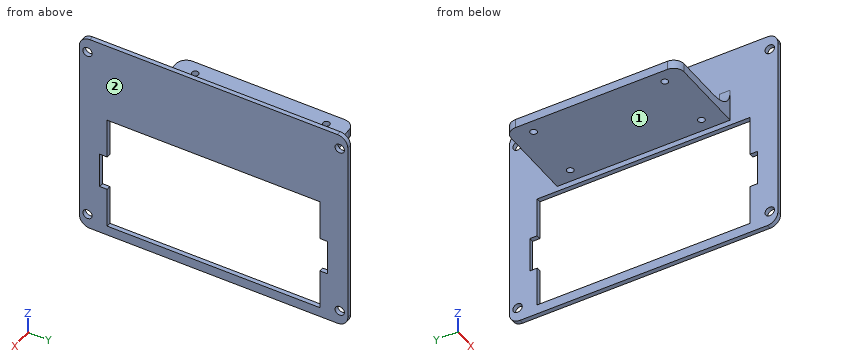
Autodesk Fusion 360 part; units mm, degrees
sketch "Sketch1" plane through (0, 0, 0) normal (1, 0, 0) x (0, 1, 0)
  line L0 (45, 35) -> (-45, 35)
  line L1 (-45, 35) -> (-45, -35)
  line L2 (-45, -35) -> (45, -35)
  line L3 (45, -35) -> (45, 35)
  line L4 (45, 35) -> (-45, -35) construction
  line L5 (-45, 35) -> (45, -35) construction
  line L6 (0, 0) -> (0, -35) construction
  line L7 (39.5, 9.4262) -> (-39.5, 9.4262) construction
  line L8 (-39.5, 9.4262) -> (-39.5, -33.5738) construction
  line L9 (-39.5, -33.5738) -> (39.5, -33.5738) construction
  line L10 (39.5, -33.5738) -> (39.5, 9.4262) construction
  line L11 (39.5, 9.4262) -> (-39.5, -33.5738) construction
  line L12 (-39.5, 9.4262) -> (39.5, -33.5738) construction
  line L13 (35.7, 7.5762) -> (-35.7, 7.5762)
  line L14 (-35.7, 7.5762) -> (-35.7, -31.7238)
  line L15 (-35.7, -31.7238) -> (35.7, -31.7238)
  line L16 (35.7, -31.7238) -> (35.7, 7.5762)
  line L17 (35.7, 7.5762) -> (-35.7, -31.7238) construction
  line L18 (-35.7, 7.5762) -> (35.7, -31.7238) construction
  circle A0 centre (42.2913, -30.0813) radius 1.575
  line L19 (0, 0) -> (10.5805, 0) construction
  circle A1 centre (-42.2913, -30.0813) radius 1.575
  circle A2 centre (42.2913, 30.0813) radius 1.575
  circle A3 centre (-42.2913, 30.0813) radius 1.575
  line L20 (0, 0) -> (0, 0.8708) construction
  line L21 (0, 0.8708) -> (0, 35) construction
  line L22 (25, 32.3854) -> (-25, 32.3854) construction
  line L23 (-25, 32.3854) -> (-25, 12.3854) construction
  line L24 (-25, 12.3854) -> (25, 12.3854) construction
  line L25 (25, 12.3854) -> (25, 32.3854) construction
  line L26 (25, 32.3854) -> (-25, 12.3854) construction
  line L27 (-25, 32.3854) -> (25, 12.3854) construction
  line L28 (29, 12.3854) -> (-29, 12.3854)
  line L29 (-29, 12.3854) -> (-29, 9.3854)
  line L30 (-29, 9.3854) -> (29, 9.3854)
  line L31 (29, 9.3854) -> (29, 12.3854)
  line L32 (29, 12.3854) -> (-29, 9.3854) construction
  line L33 (-29, 12.3854) -> (29, 9.3854) construction
  line L34 (0, -12.0738) -> (39.5, -12.0738) construction
  line L35 (35.7, -6.0738) -> (38.2, -6.0738)
  line L36 (38.2, -6.0738) -> (38.2, -18.0738)
  line L37 (38.2, -18.0738) -> (35.7, -18.0738)
  line L38 (35.7, -18.0738) -> (35.7, -6.0738)
  line L39 (-38.2, -18.0738) -> (-35.7, -18.0738)
  line L40 (-38.2, -6.0738) -> (-38.2, -18.0738)
  line L41 (-35.7, -6.0738) -> (-38.2, -6.0738)
  point P0 (0, -12.0738)
  point P1 (0, -12.0738)
  point P2 (0, 22.3854)
  point P3 (0, 10.8854)
  point P4 (38.2, -12.0738)
  dimension "d8" = 90
  dimension "d9" = 70
  dimension "d12" = 79
  dimension "d13" = 43
  dimension "d14" = 71.4
  dimension "d15" = 39.3
  dimension "d17" = 3.15
  dimension "d21" = 50
  dimension "d22" = 20
  dimension "d25" = 58
  dimension "d26" = 3
  dimension "d58" = 2.5
  dimension "d59" = 12
extrude "Extrude1" add sketch "Sketch1" along normal blind 1.5 contours L0 L1 L2 L3 | L28 L29 L30 L31
extrude "Extrude2" add sketch "Sketch1" against normal blind 29 contours L28 L29 L30 L31
sketch "Sketch2" plane through (0, 0, 12.3854) normal (0, 0, 1) x (-1, 0, 0)
  line L0 (0, 29) -> (0, -29)
  line L1 (0, -29) -> (29, -29)
  line L2 (29, -29) -> (29, 29)
  line L3 (29, 29) -> (0, 29)
  line L4 (0, 29) -> (29, -29) construction
  line L5 (27.5, 25) -> (1.5, 25) construction
  line L6 (1.5, 25) -> (1.5, -25) construction
  line L7 (1.5, -25) -> (27.5, -25) construction
  line L8 (27.5, -25) -> (27.5, 25) construction
  line L9 (27.5, 25) -> (1.5, -25) construction
  line L10 (1.5, 25) -> (27.5, -25) construction
  circle A0 centre (4.35, -22) radius 1.575 construction
  circle A1 centre (24.65, -22) radius 1.575 construction
  circle A2 centre (4.35, 22) radius 1.575 construction
  circle A3 centre (24.65, 22) radius 1.575 construction
  line L11 (4.35, -22) -> (24.65, 22) construction
  circle A4 centre (4.35, -22) radius 1.1303
  circle A5 centre (24.65, -22) radius 1.1303
  circle A6 centre (4.35, 22) radius 1.1303
  circle A7 centre (24.65, 22) radius 1.1303
  point P0 (14.5, 0)
  point P1 (14.5, 0)
  point P2 (14.5, 0)
  dimension "d32" = 26
  dimension "d33" = 50
  dimension "d37" = 3.15
  dimension "d40" = 20.3
  dimension "d41" = 44
  dimension "d51" = 2.2606
  dimension "d54" = 20.3
  dimension "d55" = 44
fillet "Fillet1" radius 3.5 2 edges at (-29, 29, 10.8854) (-29, -29, 10.8854)
fillet "Fillet2" radius 3.5 4 edges at (0.75, 45, 35) (0.75, 45, -35) (0.75, -45, 35) (0.75, -45, -35)
sketch "Sketch3" plane through (0, -29, 0) normal (0, -1, 0) x (1, 0, 0)
  line L0 (-25.5, 12.3854) -> (-25.5, 9.3854)
  line L1 (-25.5, 9.3854) -> (0, 9.3854)
  line L2 (0, 9.3854) -> (0, 12.3854)
  line L3 (0, 12.3854) -> (-25.5, 12.3854)
  line L4 (0, 35) -> (0, -35) construction
  line L5 (-27.5, 12.3854) -> (-1.5, 12.3854) construction
  spline S0 degree 5 poles (-9.6866, 12.3854) (-9.3387, 12.3854) (-8.655, 12.4012) (-7.6662, 12.4723) (-6.4221, 12.6617) (-4.9991, 13.0566) (-3.7214, 13.6129) (-2.6063, 14.3356) (-1.6713, 15.2291) (-0.9285, 16.2912) (-0.387, 17.5173) (-0.1222, 18.6267) (-0.0222, 19.5305) (0, 20.1649) (0, 20.4901) knots 0 0 0 0 0 0 0.1 0.2 0.3 0.4 0.5 0.6 0.7 0.8 0.9 1 1 1 1 1 1
  line L6 (0, 18.6225) -> (0, 22.3578)
  line L7 (-11.558, 12.3854) -> (-7.8153, 12.3854)
  line L8 (-9.6866, 12.3854) -> (0, 12.3854)
  line L9 (0, 20.4901) -> (0, 12.3854)
  point P0 (-2.4919, 14.508)
extrude "Extrude3" add sketch "Sketch3" against normal blind 3.5 contours L3 S0 L6 L7 L8 L9
sketch "Sketch4" plane through (0, 29, 0) normal (0, 1, 0) x (-1, 0, 0)
  line L0 (25.5, 9.3854) -> (25.5, 12.3854)
  line L1 (25.5, 12.3854) -> (0, 12.3854)
  line L2 (0, 12.3854) -> (0, 9.3854)
  line L3 (0, 9.3854) -> (25.5, 9.3854)
  line L4 (0, 12.3854) -> (9.6866, 12.3854)
  spline S0 degree 5 poles (9.6866, 12.3854) (9.3387, 12.3854) (8.655, 12.4012) (7.6662, 12.4723) (6.4221, 12.6617) (4.9991, 13.0566) (3.7214, 13.6129) (2.6063, 14.3356) (1.6713, 15.2291) (0.9285, 16.2912) (0.387, 17.5173) (0.1222, 18.6267) (0.0222, 19.5305) (0, 20.1649) (0, 20.4901) knots 0 0 0 0 0 0 0.1 0.2 0.3 0.4 0.5 0.6 0.7 0.8 0.9 1 1 1 1 1 1
  line L5 (0, 20.4901) -> (0, 12.3854)
extrude "Extrude4" add sketch "Sketch4" against normal blind 3.5 contours L1 L4 S0 L5
extrude "Extrude5" cut sketch "Sketch2" against normal blind 3 contours A4 | A5 | A6 | A7
equation "cutout_length = 71.4 mm"
equation "cutout_height = 39.3 mm"
equation "plastic_thick = 1.5 mm"
equation "tab_width = 12 mm"
equation "tab_thick = 2.5 mm"
equation "panel_width = 90 mm"
equation "panel_height = 70 mm"
equation "d8 = panel_width"
equation "d9 = panel_height"
equation "power_supply_width = 79 mm"
equation "power_supply_height = 43 mm"
equation "d12 = power_supply_width"
equation "d13 = power_supply_height"
equation "d14 = cutout_length"
equation "d15 = cutout_height"
equation "mount_through_hole_diam = 3.15 mm"
equation "d17 = mount_through_hole_diam"
equation "relay_height = 20 mm"
equation "relay_length = 50 mm"
equation "relay_width = 26 mm"
equation "d21 = relay_length"
equation "d22 = relay_height"
equation "relay_ledge_thick = 3 mm"
equation "relay_ledge_length = relay_length + 8 mm"
equation "d25 = relay_ledge_length"
equation "d26 = relay_ledge_thick"
equation "relay_ledge_width = relay_width + 3 mm"
equation "d28 = plastic_thick"
equation "d32 = relay_width"
equation "d33 = relay_length"
equation "relay_dist_bw_holes_length = 44 mm"
equation "relay_dist_bw_holes_width = 20.3 mm"
equation "relay_hole_diam = 3.15 mm"
equation "d37 = relay_hole_diam"
equation "d40 = relay_dist_bw_holes_width"
equation "d41 = relay_dist_bw_holes_length"
equation "relay_mount_tap_diam = 0.089 in"
equation "d51 = relay_mount_tap_diam"
equation "d54 = relay_dist_bw_holes_width"
equation "d55 = relay_dist_bw_holes_length"
equation "d58 = tab_thick"
equation "d59 = tab_width"
Here's how the part is built. I have some questions about the finished solid (model axes, mm). Face numbers are marked on the shaded views. A direction names the side the tool comes from. Round coordinates to 2 decimals unless told otherwise and drop trailing zeros. Loops run counter-clockwise (first coordinate to the right, second up) from the corner with the lowest first, then second, coordinate; pieces in that order, holes last.
1. Which directions (+Z, -Z, +X, -X, +Y, -Y) give clear straight access to the entire face, cutting with the end or side of a thin tool? Please do the marked faces 1 and 2.
Answer list:
face 1: -Z, -X, +Y, -Y
face 2: +Z, -Z, +X, +Y, -Y
2. If we section it at C-C on z = 22: Write out the boundary of the cut face in (x, y).
Answer list:
outline: (0, -45) - (1.5, -45) - (1.5, 45) - (0, 45) - close
3. If I drill on line 1 along X through (y, z) = (22, 10); line 2 along X through (y, z) = (-8.5, 19); line 3 along Z through (x, y) = (-18, 13.5), over which ranges is the centre line in solid material (lowest first)?
Answer list:
line 1: x = -29 to -25.78, -23.52 to -5.48, -3.22 to 1.5
line 2: x = 0 to 1.5
line 3: z = 9.39 to 12.39
4. If we section it at D-D on x = -4.35: Count the separate pieces of the cut face and the enclosed holes in it, plus the area to 3 significant figures.
Answer list:
separate pieces: 3
enclosed holes: 0
area: 167 mm2
5. If we section it at B-B on y = -22: Write out the boundary of the cut face in (x, z), plus the area to 3 significant figures.
Answer list:
outline: (-29, 9.39) - (-25.78, 9.39) - (-25.78, 12.39) - (-29, 12.39) - close; (-23.52, 9.39) - (-5.48, 9.39) - (-5.48, 12.39) - (-23.52, 12.39) - close; (-3.22, 9.39) - (0, 9.39) - (0, 7.58) - (1.5, 7.58) - (1.5, 35) - (0, 35) - (0, 12.39) - (-3.22, 12.39) - close; (0, -35) - (1.5, -35) - (1.5, -31.72) - (0, -31.72) - close
area: 119 mm2
6. If we section it at A-A on y = 9.5: Write out the boundary of the cut face in (x, z).
Answer list:
outline: (-29, 9.39) - (0, 9.39) - (0, 7.58) - (1.5, 7.58) - (1.5, 35) - (0, 35) - (0, 12.39) - (-29, 12.39) - close; (0, -35) - (1.5, -35) - (1.5, -31.72) - (0, -31.72) - close
7. For P1, Ø6.5, axis at x = -4.5, z = 14.5, coming from the +Y side; P2, Ø12, axis at y = 20, z = 0, coming from the -X side; P3, Ø3, axis at x = -4.35, y = -22, coming from the -Z side; P4, Ø2.5, axis at x = -4.35, y = 22, coming from the +Z side, each with a flat end and sliding along its axis, tell me the tip position at first contact or that it passes through.
Answer list:
P1: stops at y = 29
P2: passes through
P3: stops at z = 9.39
P4: stops at z = 12.39
